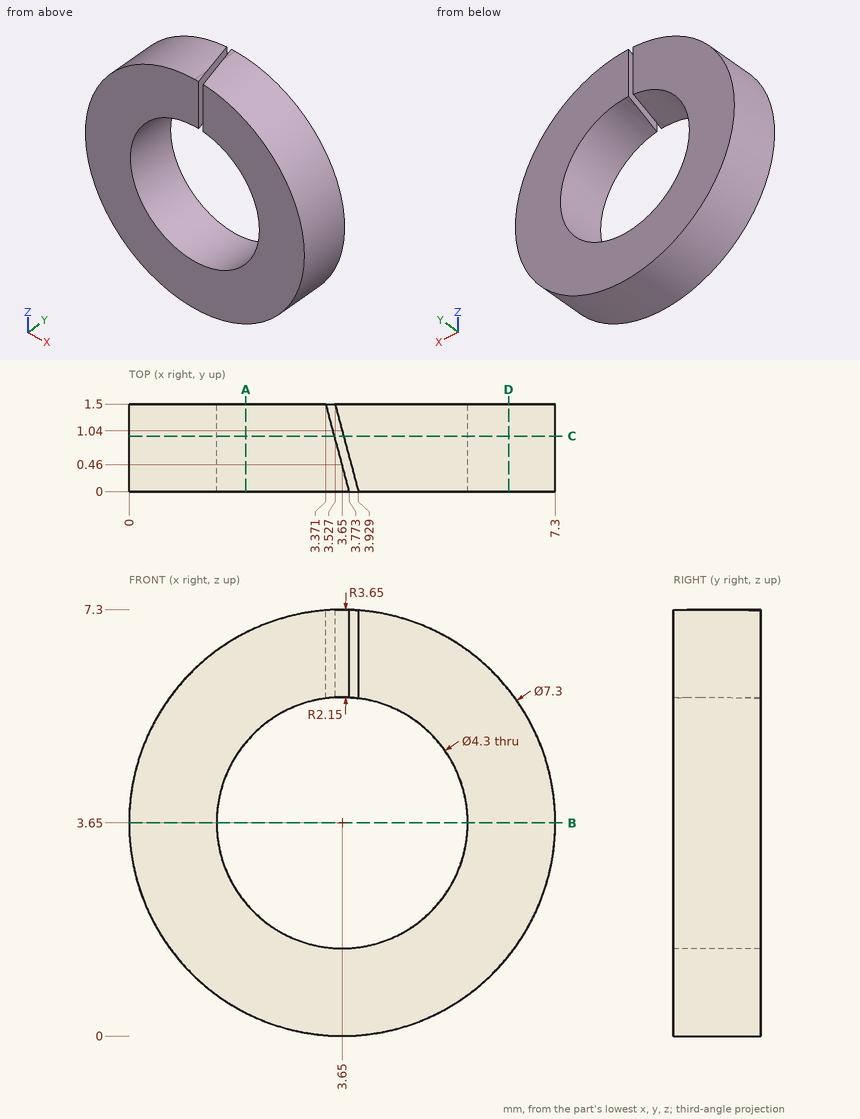
Source: three-view drawing plus pictorial views. Frame: mm from the lowest corner of the part. Round coordinates to 2 decimals unless told otherwise and drop trailing zeros. Write each loop counter-clockwise with the first axis right and the second up, starting at its lowest first coordinate (ties: lowest second). Pieces come first, ordered by that corner, then holes. Notation, with made-up numbers: M -3,6 L 23,6 A20 cw 23,39 Z; hole C 14.25,-26.75 d7. An arc over 180 degrees is marked long. One line per item, written item: value. Start each with the question number.
Item 1: Section query A-A (x = 2). Return the cut outline in (y, z) (1 decimal).
Item 2: Section query C-C (y = 0.95). Return the cut outline in (x, z), plus the area to 3 significant figures.
Item 3: Ray query, L1, parallel to X at y = 1, z = 3.65; L2, parallel to X at y = 0.9, z = 6; L3, parallel to Z at x = 4, y = 0.3. Return the intervals inside material, ascending. Write a range as from..to.
Item 4: Section query D-D (x = 6.5). Return the cut outline in (y, z).
Item 5: Section query B-B (z = 3.65). Return the cut outline in (x, y).
Result set:
1. outline: M 0,0.4 L 1.5,0.4 L 1.5,2.3 L 0,2.3 Z; M 0,5 L 1.5,5 L 1.5,6.9 L 0,6.9 Z
2. outline: M 3.52,5.8 L 3.52,7.3 A3.65 ccw long 3.67,7.3 L 3.67,5.8 A2.15 cw long Z
2. area: 27.1 mm²
3. L1: x = 0..1.5, 5.8..7.3
3. L2: x = 0.86..3.53, 3.69..6.44
3. L3: z = 0.02..1.53, 5.77..7.28
4. outline: M 0,1.37 L 1.5,1.37 L 1.5,5.93 L 0,5.93 Z
5. outline: M 0,0 L 1.5,0 L 1.5,1.5 L 0,1.5 Z; M 5.8,0 L 7.3,0 L 7.3,1.5 L 5.8,1.5 Z
